Work out the finished part from the listing and answer in its coordinate system (mm). Face numbers are marked on the shaded views. A direction names the side the tool comes from. Coordinates: 2 decimals unless noted, no trailing zeros. Loops run counter-clockwise (first coordinate to the right, second up) from the corner with the lowest first, then second, coordinate; pieces in that order, holes last. Notation, with made-up numbers: (71.25, -34) - (77.25, -34) arc R29 ccw to (77.25, -5) - close; hole circle Ø7 at (57, -35.5). An arc over 180 degrees is marked (long way). Write each question's results on one line, items separated by ' | '. Start each with the question number.
1. Which of the six approach directions +Z, -Z, +X, -X, +Y, -Y give full straight-line access (tool end or side, diameter ignored) to the marked faces 1, 2, 3 and 4?
2. A cutting plane is placed at C-C on x = 0. Determine the outline of the cut face in (y, z), then the cut area to 3 significant figures.
3. Each of these flat-tipped pins is pushed along its axis until it touches: P1, Ø3, axis at x = -2, y = -5, coming from the +Z side; P2, Ø2, axis at y = -0.5, z = -3, coming from the -X side; P3, Ø4.5, axis at x = 1, y = -19, coming from the -Z side. Where does it stop, or does it pass through?
4. A cutting plane is placed at A-A on y = -12. Determine the outline of the cut face in (x, z), then the cut area to 3 significant figures.
5. A cutting plane is placed at D-D on x = -4.25. State how many separate pieces and enclosed holes the cut face has, then the cut area to 3 significant figures.
6. Find the intervals of material crossed by line 1 along Y through (x, z) = (-5, 0.5); line 2 along Z through (x, y) = (2, -28.5); line 3 along Y through (x, z) = (-0.75, -7.75), in increasing order. Write a range as [from, to].
7. A cutting plane is placed at B-B on z = 0. Determine the outline of the cut face in (x, y), then the cut area to 3 significant figures.
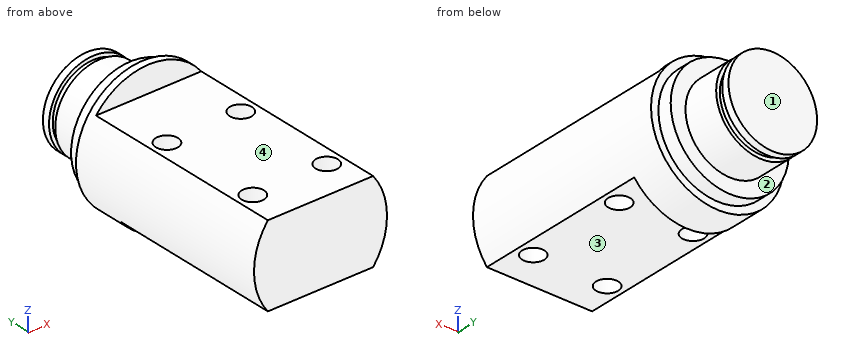
from build123d import *

# Parameters (mm, degrees)
SKETCH_1_R          = 6
EXTRUDE_1_DEPTH     = 7
SKETCH_2_R          = 9
EXTRUDE_2_DEPTH     = 31
SKETCH_3_W          = 19.613357353
SKETCH_3_H          = 3.5
CUT_EXTRUDE_1_DEPTH = 24
SKETCH_4_W          = 20.018720859
SKETCH_4_H          = 3.5
CUT_EXTRUDE_2_DEPTH = 28
SKETCH_5_R          = 1.5
CUT_EXTRUDE_3_DEPTH = 18
SKETCH_11_R         = 10.638163441
SKETCH_11_R_2       = 5.5
CUT_EXTRUDE_4_DEPTH = 1
SKETCH_12_R         = 9
SKETCH_12_R_2       = 8
CUT_EXTRUDE_7_DEPTH = 2


with BuildPart() as part:
    # 草图1 → 凸台-拉伸1 (new body)
    with BuildSketch(Plane(origin=(0, 0, 0), x_dir=(1, 0, 0), z_dir=(0, 1, 0))):
        Circle(SKETCH_1_R)
    extrude(amount=EXTRUDE_1_DEPTH)

    # 草图2 → 凸台-拉伸2 (add)
    with BuildSketch(Plane.XZ):
        Circle(SKETCH_2_R)
    extrude(amount=EXTRUDE_2_DEPTH)

    # 草图3 → 切除-拉伸1 (cut)
    with BuildSketch(Plane.XZ.offset(31)):
        with Locations((1.075772383, -7.25)):
            Rectangle(SKETCH_3_W, SKETCH_3_H)
    extrude(amount=-CUT_EXTRUDE_1_DEPTH, mode=Mode.SUBTRACT)

    # 草图4 → 切除-拉伸2 (cut)
    with BuildSketch(Plane.XZ.offset(31)):
        with Locations((1.37199956, 7.25)):
            Rectangle(SKETCH_4_W, SKETCH_4_H)
    extrude(amount=-CUT_EXTRUDE_2_DEPTH, mode=Mode.SUBTRACT)

    # 草图5 → 切除-拉伸3 (cut)
    with BuildSketch(Plane(origin=(0, 0, -5.5), x_dir=(-1, 0, 0), z_dir=(0, 0, -1))):
        with Locations((-5, -26)):
            Circle(SKETCH_5_R)
        with Locations((5, -26)):
            Circle(SKETCH_5_R)
        with Locations((5, -12)):
            Circle(SKETCH_5_R)
        with Locations((-5, -12)):
            Circle(SKETCH_5_R)
    extrude(amount=-CUT_EXTRUDE_3_DEPTH, mode=Mode.SUBTRACT)

    # 草图11 → 切除-拉伸4 (cut)
    with BuildSketch(Plane(origin=(0, 6, 0), x_dir=(1, 0, 0), z_dir=(0, 1, 0))):
        Circle(SKETCH_11_R)
        Circle(SKETCH_11_R_2, mode=Mode.SUBTRACT)
    extrude(amount=-CUT_EXTRUDE_4_DEPTH, mode=Mode.SUBTRACT)

    # 草图12 → 切除-拉伸7 (cut)
    with BuildSketch(Plane(origin=(0, 0, 0), x_dir=(1, 0, 0), z_dir=(0, 1, 0))):
        Circle(SKETCH_12_R)
        Circle(SKETCH_12_R_2, mode=Mode.SUBTRACT)
    extrude(amount=-CUT_EXTRUDE_7_DEPTH, mode=Mode.SUBTRACT)


solid = part.part
Values:
1) face 1: +Z, -Z, +X, -X, +Y | face 2: +Y | face 3: -Z, +X, -X, -Y | face 4: +Z, +X, -X, -Y
2) outline: (-31, -5.5) - (-7, -5.5) - (-7, -9) - (-2, -9) - (-2, -8) - (0, -8) - (0, -6) - (5, -6) - (5, -5.5) - (6, -5.5) - (6, -6) - (7, -6) - (7, 6) - (6, 6) - (6, 5.5) - (5, 5.5) - (5, 6) - (0, 6) - (0, 8) - (-2, 8) - (-2, 9) - (-3, 9) - (-3, 5.5) - (-31, 5.5) - close | area: 455 mm^2
3) P1: z = 5.5 | P2: x = -7.75 | P3: z = -5.5
4) outline: (-7.12, -5.5) - (-6.5, -5.5) - (-6.5, 5.5) - (-7.12, 5.5) arc R9 ccw to start; (-3.5, -5.5) - (3.5, -5.5) - (3.5, 5.5) - (-3.5, 5.5) - close; (6.5, -5.5) - (7.12, -5.5) arc R9 ccw to (7.12, 5.5) - (6.5, 5.5) - close | area: 119 mm^2
5) separate pieces: 3 | enclosed holes: 0 | area: 361 mm^2
6) line 1: [-31, -27.5], [-24.5, -13.5], [-10.5, 7] | line 2: [-5.5, 5.5] | line 3: [-7, 0]
7) outline: (-9, -31) - (9, -31) - (9, -2) - (8, -2) - (8, 0) - (6, 0) - (6, 5) - (5.5, 5) - (5.5, 6) - (6, 6) - (6, 7) - (-6, 7) - (-6, 6) - (-5.5, 6) - (-5.5, 5) - (-6, 5) - (-6, 0) - (-8, 0) - (-8, -2) - (-9, -2) - close; hole circle Ø3 at (-5, -26); hole circle Ø3 at (-5, -12); hole circle Ø3 at (5, -26); hole circle Ø3 at (5, -12) | area: 609 mm^2
